The listing builds one solid part. Answer for the finished solid, in the listing's coordinates (mm). A direction names the side the tool comes from. Round coordinates to 2 decimals unless told otherwise and drop trailing zeros. Order: outer loops, then holes, each group sorted by start corner. A loop starts at its lowest first (then second) coordinate and runs counter-clockwise, first axis right, second up. Notation, with made-up numbers: M 19,-36.75 L 71,-36.75 A21 cw 71,1.25 Z; hole C 4,28 d7. An arc over 180 degrees is marked long. Write item = value, one per line. Start each with the question number.
(1) A cutting plane is placed at D-D, the plane z = 2.5. Determine the outline of the cut face in (x, y).
(2) Straight lines are drawn through the part: probe 1 along Y at (x, z) = (12.3, 0); probe 2 along Y at (x, z) = (12, 1.25); probe 3 along X at (y, z) = (31, -5.75). For each, find the intervals that lie inside material, in ascending order. Write a range as from..to.
(3) Each of these flat-tipped pins is pushed along its axis until it touches: pin 1 (1.5 mm diameter, centred on x = 14.5, z = -6.5, fed in from +Y); pin 2 (1.5 mm diameter, centred on x = 11, z = 3, fed in from +Y); pin 3 (1 mm diameter, centred on x = 11.5, z = -4, fed in from -Y). Where does it stop, or does it pass through?
(4) Which of the six approach directions +Z, -Z, +X, -X, +Y, -Y give full straight-line access (tool end or side, diameter ignored) to faces 1 (the face through (13, 9.4, -7)), 2 (the face through (11, 3.8, 0)), 3 (the face through (13, -33.4, -7)), 4 (the face through (13, 8, 5.4)), 5 (the face through (11, -12, -7))?
(5) For a pull along Z with two mould halves and no side action, classify faces 6 (the face through (5, 0, -10)), 7 (the face through (13, -12, 0)), 8 (the face through (11.4, 0, 0)), 9 (the face through (11, -12, 7)) as released by +Z, released by -Z, zero draft, split by the parting line, or undercut.
(6) A cutting plane is placed at C-C, the plane y = -9.5. Determine the outline of the cut face in (x, z), and give its area (3 significant figures).
(7) A cutting plane is placed at A-A, the plane y = -23.5. Determine the outline of the cut face in (x, z).
(8) A cutting plane is placed at B-B, the plane z = -0.25. Determine the outline of the cut face in (x, y), and give its area (3 significant figures).
from build123d import *

# Parameters (mm, degrees)
SKETCH1_W           = 20
SKETCH1_H           = 70
BOSS_EXTRUDE1_DEPTH = 10
SKETCH2_W           = 3
SKETCH2_H           = 3
BOSS_EXTRUDE2_DEPTH = 7
SKETCH3_W           = 14
SKETCH3_H           = 31.6
BOSS_EXTRUDE3_DEPTH = 3
SKETCH4_R           = 3.25
CUT_EXTRUDE1_DEPTH  = 1.6


with BuildPart() as part:
    # Sketch1 → Boss-Extrude1 (new body)
    with BuildSketch(Plane(origin=(0, 0, 0), x_dir=(0, 0, -1), z_dir=(1, 0, 0))):
        Rectangle(SKETCH1_W, SKETCH1_H)
    extrude(amount=BOSS_EXTRUDE1_DEPTH)

    # Sketch2 → Boss-Extrude2 (add)
    with BuildSketch(Plane(origin=(10, 0, 0), x_dir=(0, 0, -1), z_dir=(1, 0, 0))):
        with Locations((-6.9, 7.9)):
            Rectangle(SKETCH2_W, SKETCH2_H)
        with Locations((6.9, 7.9)):
            Rectangle(SKETCH2_W, SKETCH2_H)
        with Locations((6.9, -31.9)):
            Rectangle(SKETCH2_W, SKETCH2_H)
        with Locations((-6.9, -31.9)):
            Rectangle(SKETCH2_W, SKETCH2_H)
    extrude(amount=BOSS_EXTRUDE2_DEPTH)

    # Sketch3 → Boss-Extrude3 (add)
    with BuildSketch(Plane(origin=(10, 0, 0), x_dir=(0, 0, -1), z_dir=(1, 0, 0))):
        with Locations((0, -12)):
            Rectangle(SKETCH3_W, SKETCH3_H)
    extrude(amount=BOSS_EXTRUDE3_DEPTH)

    # Sketch4 → Cut-Extrude1 (cut)
    with BuildSketch(Plane(origin=(13, 0, 0), x_dir=(0, 0, -1), z_dir=(1, 0, 0))):
        with Locations((0, -23.5)):
            Circle(SKETCH4_R)
        with Locations((0, -0.5)):
            Circle(SKETCH4_R)
    extrude(amount=-CUT_EXTRUDE1_DEPTH, mode=Mode.SUBTRACT)


solid = part.part
Reported:
q1.outline = M 0,-35 L 10,-35 L 10,-27.8 L 13,-27.8 L 13,-25.58 L 11.4,-25.58 L 11.4,-21.42 L 13,-21.42 L 13,-2.58 L 11.4,-2.58 L 11.4,1.58 L 13,1.58 L 13,3.8 L 10,3.8 L 10,35 L 0,35 Z
q2.probe_1 = -27.8..-26.75, -20.25..-3.75, 2.75..3.8
q2.probe_2 = -27.8..-26.5, -20.5..-3.5, 2.5..3.8
q2.probe_3 = 0..10
q3.pin_1 = 9.4
q3.pin_2 = 3.8
q3.pin_3 = -27.8
q4.face_1 = +Z, -Z, +X, +Y
q4.face_2 = +Z, -Z, +X
q4.face_3 = +Z, -Z, +X, -Y
q4.face_4 = +X, +Y
q4.face_5 = -Z, +X
q5.face_6 = released by -Z
q5.face_7 = zero draft
q5.face_8 = undercut
q5.face_9 = released by +Z
q6.outline = M 0,-10 L 10,-10 L 10,-7 L 13,-7 L 13,7 L 10,7 L 10,10 L 0,10 Z
q6.area = 242 mm²
q7.outline = M 0,-10 L 10,-10 L 10,-7 L 13,-7 L 13,-3.25 L 11.4,-3.25 L 11.4,3.25 L 13,3.25 L 13,7 L 10,7 L 10,10 L 0,10 Z
q8.outline = M 0,-35 L 10,-35 L 10,-27.8 L 13,-27.8 L 13,-26.74 L 11.4,-26.74 L 11.4,-20.26 L 13,-20.26 L 13,-3.74 L 11.4,-3.74 L 11.4,2.74 L 13,2.74 L 13,3.8 L 10,3.8 L 10,35 L 0,35 Z
q8.area = 774 mm²
